```python
from build123d import *

# Parameters (mm, degrees)
SKETCH1_W                                    = 95.25
SKETCH1_H                                    = 82.55
BOSS_EXTRUDE1_DEPTH                          = 3.175
SKETCH2_W                                    = 95.25
SKETCH2_H                                    = 82.55
SKETCH2_W_2                                  = 88.9
SKETCH2_H_2                                  = 76.2
BOSS_EXTRUDE2_DEPTH                          = 28.9
SKETCH3_W                                    = 91.821
SKETCH3_H                                    = 79.121
SKETCH3_W_2                                  = 88.9
SKETCH3_H_2                                  = 76.2
BOSS_EXTRUDE3_DEPTH                          = 1.5875
FILLET1_R                                    = 1.5875
SKETCH4_R                                    = 1.7018
CUT_EXTRUDE1_DEPTH                           = 72.448793945
CUT_EXTRUDE2_DEPTH                           = 2.35
BOSS_EXTRUDE4_START                          = 19.05
SKETCH7_R                                    = 3.175
SKETCH7_R_2                                  = 1.7145
BOSS_EXTRUDE4_DEPTH                          = 19.05
SKETCH8_R                                    = 1.7145
CUT_EXTRUDE3_DEPTH                           = 67.826019446
MIRROR1_START                                = 19.05
MIRROR1_AT_THE_SECOND_PLANE_COPY_1_SKETC_R   = 3.175
MIRROR1_AT_THE_SECOND_PLANE_COPY_1_SKETC_R_2 = 1.7145
MIRROR1_AT_THE_SECOND_PLANE_COPY_1_DEPTH     = 19.05
MIRROR1_AT_THE_SECOND_PLANE_COPY_2_SKETC_R   = 1.7145
MIRROR1_AT_THE_SECOND_PLANE_COPY_2_DEPTH     = 67.826019446
CUT_EXTRUDE4_DEPTH                           = 2.4
MIRROR2_AT_THE_SECOND_PLANE_COPY_1_DEPTH     = 2.4
CUT_EXTRUDE5_DEPTH                           = 107.370085815


with BuildPart() as part:
    # Sketch1 → Boss-Extrude1 (new body)
    with BuildSketch(Plane.XY):
        Rectangle(SKETCH1_W, SKETCH1_H)
    extrude(amount=BOSS_EXTRUDE1_DEPTH)

    # Sketch2 → Boss-Extrude2 (add)
    with BuildSketch(Plane.XY.offset(3.175)):
        Rectangle(SKETCH2_W, SKETCH2_H)
        Rectangle(SKETCH2_W_2, SKETCH2_H_2, mode=Mode.SUBTRACT)
    extrude(amount=BOSS_EXTRUDE2_DEPTH)

    # Sketch3 → Boss-Extrude3 (add)
    with BuildSketch(Plane.XY.offset(32.075)):
        Rectangle(SKETCH3_W, SKETCH3_H)
        Rectangle(SKETCH3_W_2, SKETCH3_H_2, mode=Mode.SUBTRACT)
    extrude(amount=BOSS_EXTRUDE3_DEPTH)

    # Fillet1
    fillet1_edges = [part.edges().sort_by_distance(p)[0] for p in [
        (44.45, 38.1, 18.41875),
        (-44.45, 38.1, 18.41875),
        (-44.45, -38.1, 18.41875),
        (44.45, -38.1, 18.41875),
        (45.9105, -39.5605, 32.86875),
        (45.9105, 39.5605, 32.86875),
        (-45.9105, 39.5605, 32.86875),
        (-45.9105, -39.5605, 32.86875),
        (47.625, -41.275, 16.0375),
        (-47.625, -41.275, 16.0375),
        (-47.625, 41.275, 16.0375),
        (47.625, 41.275, 16.0375),
    ]]
    fillet(fillet1_edges, radius=FILLET1_R)

    # Sketch4 → Cut-Extrude1 (cut, through all)
    with BuildSketch(Plane(origin=(0, 0, 0), x_dir=(-1, 0, 0), z_dir=(0, 0, -1))):
        with Locations((0, 21.749999934)):
            Circle(SKETCH4_R)
        with Locations((0, -21.749999934)):
            Circle(SKETCH4_R)
    extrude(amount=-CUT_EXTRUDE1_DEPTH, mode=Mode.SUBTRACT)

    # Sketch5 → Cut-Extrude2 (cut)
    with BuildSketch(Plane(origin=(0, 0, 0), x_dir=(-1, 0, 0), z_dir=(0, 0, -1))):
        Polygon((3.446203757, 21.749999934), (1.723101878, 24.734499934), (-1.723101878, 24.734499934), (-3.446203757, 21.749999934), (-1.723101878, 18.765499934), (1.723101878, 18.765499934), align=None)
        Polygon((1.723101878, -18.765499934), (3.446203757, -21.749999934), (1.723101878, -24.734499934), (-1.723101878, -24.734499934), (-3.446203757, -21.749999934), (-1.723101878, -18.765499934), align=None)
    extrude(amount=-CUT_EXTRUDE2_DEPTH, mode=Mode.SUBTRACT)

    # Sketch7 → Boss-Extrude4 (add)
    # profile 1 of 4: a face of its own
    with BuildSketch(Plane.XY.offset(3.175).offset(BOSS_EXTRUDE4_START)):
        with BuildLine():
            ThreePointArc((-44.45, 34.925), (-43.520064053, 37.170064008), (-41.275000064, 38.1))
            Line((-41.275000064, 38.1), (-42.8625, 38.1))
            ThreePointArc((-42.8625, 38.1), (-43.985032015, 37.635032015), (-44.45, 36.5125))
            Line((-44.45, 36.5125), (-44.45, 34.925))
        make_face()
    # profile 2 of 4: a face of its own
    with BuildSketch(Plane.XY.offset(3.175).offset(BOSS_EXTRUDE4_START)):
        with BuildLine():
            Line((-44.45, 34.925), (-44.45, 31.75))
            Line((-44.45, 31.75), (-41.275, 31.75))
            ThreePointArc((-41.275, 31.75), (-43.52006403, 32.67993597), (-44.45, 34.925))
        make_face()
    # profile 3 of 4: a face of its own
    with BuildSketch(Plane.XY.offset(3.175).offset(BOSS_EXTRUDE4_START)):
        with BuildLine():
            Line((-38.1, 34.925), (-38.1, 38.1))
            Line((-38.1, 38.1), (-41.275000064, 38.1))
            ThreePointArc((-41.275000064, 38.1), (-39.029935992, 37.170064053), (-38.1, 34.925))
        make_face()
    # profile 4 of 4: a face of its own
    with BuildSketch(Plane.XY.offset(3.175).offset(BOSS_EXTRUDE4_START)):
        with Locations((-41.275, 34.925)):
            Circle(SKETCH7_R)
        with Locations(Location((-41.275, 34.925, 0), (0, 0, 180))):
            Circle(SKETCH7_R_2, mode=Mode.SUBTRACT)
    boss_extrude4 = extrude(amount=-BOSS_EXTRUDE4_DEPTH)

    # Sketch8 → Cut-Extrude3 (cut, through all)
    with BuildSketch(Plane.XY.offset(22.225)):
        with Locations(Location((-41.275, 34.925, 0), (0, 0, 180))):
            Circle(SKETCH8_R)
    cut_extrude3 = extrude(amount=-CUT_EXTRUDE3_DEPTH, mode=Mode.SUBTRACT)

    # Mirror1: Boss-Extrude4, Cut-Extrude3 across plane
    add(boss_extrude4.mirror(Plane(origin=(0, 0, 0), x_dir=(0, 0, 1), z_dir=(1, 0, 0))))
    add(cut_extrude3.mirror(Plane(origin=(0, 0, 0), x_dir=(0, 0, 1), z_dir=(1, 0, 0))), mode=Mode.SUBTRACT)

    # Mirror1 at the second plane: Boss-Extrude4, Cut-Extrude3 across plane
    add(boss_extrude4.mirror(Plane.ZX))
    add(cut_extrude3.mirror(Plane.ZX), mode=Mode.SUBTRACT)

    # Mirror1 at the second plane copy 1 sketc → Mirror1 at the second plane copy 1 (add)
    # profile 1 of 4: a face of its own
    with BuildSketch(Plane(origin=(0, 0, 3.175), x_dir=(-1, 0, 0), z_dir=(0, 0, 1)).offset(MIRROR1_START)):
        with BuildLine():
            ThreePointArc((-44.45, 34.925), (-43.520064053, 37.170064008), (-41.275000064, 38.1))
            Line((-41.275000064, 38.1), (-42.8625, 38.1))
            ThreePointArc((-42.8625, 38.1), (-43.985032015, 37.635032015), (-44.45, 36.5125))
            Line((-44.45, 36.5125), (-44.45, 34.925))
        make_face()
    # profile 2 of 4: a face of its own
    with BuildSketch(Plane(origin=(0, 0, 3.175), x_dir=(-1, 0, 0), z_dir=(0, 0, 1)).offset(MIRROR1_START)):
        with BuildLine():
            Line((-44.45, 34.925), (-44.45, 31.75))
            Line((-44.45, 31.75), (-41.275, 31.75))
            ThreePointArc((-41.275, 31.75), (-43.52006403, 32.67993597), (-44.45, 34.925))
        make_face()
    # profile 3 of 4: a face of its own
    with BuildSketch(Plane(origin=(0, 0, 3.175), x_dir=(-1, 0, 0), z_dir=(0, 0, 1)).offset(MIRROR1_START)):
        with BuildLine():
            Line((-38.1, 34.925), (-38.1, 38.1))
            Line((-38.1, 38.1), (-41.275000064, 38.1))
            ThreePointArc((-41.275000064, 38.1), (-39.029935992, 37.170064053), (-38.1, 34.925))
        make_face()
    # profile 4 of 4: a face of its own
    with BuildSketch(Plane(origin=(0, 0, 3.175), x_dir=(-1, 0, 0), z_dir=(0, 0, 1)).offset(MIRROR1_START)):
        with Locations((-41.275, 34.925)):
            Circle(MIRROR1_AT_THE_SECOND_PLANE_COPY_1_SKETC_R)
        with Locations(Location((-41.275, 34.925, 0), (0, 0, 180))):
            Circle(MIRROR1_AT_THE_SECOND_PLANE_COPY_1_SKETC_R_2, mode=Mode.SUBTRACT)
    extrude(amount=-MIRROR1_AT_THE_SECOND_PLANE_COPY_1_DEPTH)

    # Mirror1 at the second plane copy 2 sketc → Mirror1 at the second plane copy 2 (cut, through all)
    with BuildSketch(Plane(origin=(0, 0, 22.225), x_dir=(-1, 0, 0), z_dir=(0, 0, 1))):
        with Locations(Location((-41.275, 34.925, 0), (0, 0, 180))):
            Circle(MIRROR1_AT_THE_SECOND_PLANE_COPY_2_SKETC_R)
    extrude(amount=-MIRROR1_AT_THE_SECOND_PLANE_COPY_2_DEPTH, mode=Mode.SUBTRACT)

    # Sketch9 → Cut-Extrude4 (cut)
    with BuildSketch(Plane(origin=(0, 0, 0), x_dir=(-1, 0, 0), z_dir=(0, 0, -1))):
        Polygon((-37.828218894, 34.925), (-39.551609447, 37.909999999), (-42.998390553, 37.909999999), (-44.721781106, 34.925), (-42.998390553, 31.940000001), (-39.551609447, 31.940000001), align=None)
    cut_extrude4 = extrude(amount=-CUT_EXTRUDE4_DEPTH, mode=Mode.SUBTRACT)

    # Mirror2: Cut-Extrude4 across plane
    add(cut_extrude4.mirror(Plane(origin=(0, 0, 0), x_dir=(0, 0, 1), z_dir=(1, 0, 0))), mode=Mode.SUBTRACT)

    # Mirror2 at the second plane: Cut-Extrude4 across plane
    add(cut_extrude4.mirror(Plane.ZX), mode=Mode.SUBTRACT)

    # Mirror2 at the second plane copy 1 sketc → Mirror2 at the second plane copy 1 (cut)
    with BuildSketch(Plane(origin=(0, 0, 0), x_dir=(1, 0, 0), z_dir=(0, 0, -1))):
        Polygon((-37.828218894, 34.925), (-39.551609447, 37.909999999), (-42.998390553, 37.909999999), (-44.721781106, 34.925), (-42.998390553, 31.940000001), (-39.551609447, 31.940000001), align=None)
    extrude(amount=-MIRROR2_AT_THE_SECOND_PLANE_COPY_1_DEPTH, mode=Mode.SUBTRACT)

    # Sketch10 → Cut-Extrude5 (cut, through all)
    with BuildSketch(Plane(origin=(-44.45, 0, 0), x_dir=(0, 0, -1), z_dir=(1, 0, 0))):
        with BuildLine():
            ThreePointArc((-20.00625, 0), (-18.41875, -1.5875), (-16.83125, 0))
            Line((-16.83125, 0), (-20.00625, 0))
        make_face()
        with BuildLine():
            Line((-20.00625, 0), (-16.83125, 0))
            ThreePointArc((-16.83125, 0), (-18.41875, 1.5875), (-20.00625, 0))
        make_face()
    extrude(amount=-CUT_EXTRUDE5_DEPTH, mode=Mode.SUBTRACT)


solid = part.part
```
For this review, take the finished solid that the model builds, in its own axes (mm). A direction names the side the tool comes from. Round coordinates to 2 decimals unless told otherwise and drop trailing zeros. Answer as a JSON object with one key per item and string values.
1. For pin 1 Ø1.3 at (y, z) = (17, 33) entering from -X; pin 2 Ø1 at (x, y) = (22.5, -28.5) entering from -Z; pin 3 Ø5.5 at (x, y) = (-41.275, -34.925) entering from +Z (3 decimals); pin 4 Ø0.5 at (y, z) = (13, 32.5) entering from +X, all flat-tipped, find the tip position at first contact; note any pin that passes through.
Response values:
{"pin 1": "stops at x = -45.91", "pin 2": "stops at z = 0", "pin 3": "stops at z = 22.225", "pin 4": "stops at x = 45.91"}
2. Tool access review of faces 1 (the face through (-0.915, 23.185, 2.757)), 2 (the face through (-1, -38.1, 18)), 3 (the face through (-1.5, 23.1, 2.35)): name each direction out of +Z, -Z, +X, -X, +Y, -Y from which nothing blocks a thin tool from reaching the whole face with its end or side.
Response values:
{"face 1": "+Z, -Z", "face 2": "+Z", "face 3": "-Z"}
3. To check wall thickness, follow line 1 along Y through (x, z) = (0, 2) (1 decimal); line 2 along X through (y, z) = (25.5, 8.5) (3 decimals); line 3 along Y through (x, z) = (23, 8.5) (3 decimals). State the ranges of each line that lie inside material, in increasing order.
Response values:
{"line 1": "y = -41.3 to -24.7, -18.8 to 18.8, 24.7 to 41.3", "line 2": "x = -47.625 to -44.45, 44.45 to 47.625", "line 3": "y = -41.275 to -38.1, 38.1 to 41.275"}
4. We need section A-A on x = 0. Count the separate pieces of the cut face and the enclosed holes in it, then the cut area to 3 significant figures.
Response values:
{"separate pieces": "3", "enclosed holes": "0", "area": "417 mm2"}
